Build history of the part. All positions in model axes, mm. Face numbers are marked on the shaded views. A direction names the side the tool comes from. Round coordinates to 2 decimals unless told otherwise and drop trailing zeros. Write each loop counter-clockwise with the first axis right and the second up, starting at its lowest first coordinate (ties: lowest second). Pieces come first, ordered by that corner, then holes. Notation, with made-up numbers: (-8, 17) -> (18, 17) arc R11 cw to (18, 31) -> close; hole circle Ø7 at (84, 26). An arc over 180 degrees is marked (long way). Return JSON: item names as keys, results as strings.
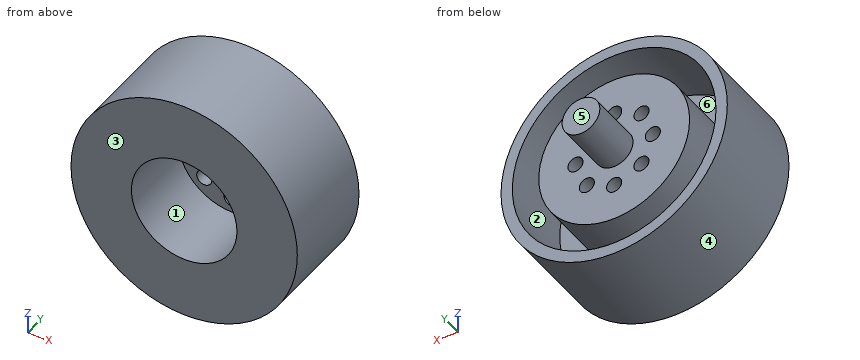
from build123d import *

# Parameters (mm, degrees)
F0_R      = 19.05
F1_DEPTH  = 16.51
F2_R      = 8.89
F4_DEPTH  = 12.7
F3_R      = 1.27
F5_DEPTH  = 25.4
F6_R      = 3.175
F7_DEPTH  = 12.7
F8_R      = 4.445
F9_DEPTH  = 0.635
F10_R     = 1.27
F11_DEPTH = 2.54
F12_R     = 0.508
F13_DEPTH = 1.016
F14_R     = 17.145
F14_R_2   = 12.7
F15_DEPTH = 12.7


with BuildPart() as f1:
    # F0 (on Front) → F1 (new body)
    with BuildSketch(Plane.XZ):
        Circle(F0_R)
    extrude(amount=-F1_DEPTH)

    # F2 (on face) → F4 (cut)
    with BuildSketch(Plane.XZ):
        Circle(F2_R)
    extrude(amount=-F4_DEPTH, mode=Mode.SUBTRACT)

    # F3 (on face) → F5 (cut)
    with BuildSketch(Plane.XZ):
        with Locations((0, 6.510976)):
            Circle(F3_R)
        with Locations((4.603955, 4.603955)):
            Circle(F3_R)
        with Locations((6.510976, 0)):
            Circle(F3_R)
        with Locations((4.603955, -4.603955)):
            Circle(F3_R)
        with Locations((0, -6.510976)):
            Circle(F3_R)
        with Locations((-4.603955, -4.603955)):
            Circle(F3_R)
        with Locations((-6.510976, 0)):
            Circle(F3_R)
        with Locations((-4.603955, 4.603955)):
            Circle(F3_R)
    extrude(amount=-F5_DEPTH, mode=Mode.SUBTRACT)

    # F6 (on face) → F7 (join)
    with BuildSketch(Plane.XZ.offset(-12.7)):
        Circle(F6_R)
    extrude(amount=-F7_DEPTH)

    # F8 (on face) → F9 (join)
    with BuildSketch(Plane.XZ.offset(-12.7)):
        Circle(F8_R)
    extrude(amount=F9_DEPTH)

    # F10 (on face) → F11 (join)
    with BuildSketch(Plane.XZ.offset(-12.065)):
        Circle(F10_R)
    extrude(amount=F11_DEPTH)

    # F12 (on face) → F13 (join)
    with BuildSketch(Plane.XZ.offset(-12.065)):
        with Locations((1.77372, 2.441316)):
            Circle(F12_R)
        with Locations((2.869939, 0.9325)):
            Circle(F12_R)
        with Locations((2.869939, -0.9325)):
            Circle(F12_R)
        with Locations((1.77372, -2.441316)):
            Circle(F12_R)
        with Locations((0, -3.017632)):
            Circle(F12_R)
        with Locations((-1.77372, -2.441316)):
            Circle(F12_R)
        with Locations((-2.869939, -0.9325)):
            Circle(F12_R)
        with Locations((-2.869939, 0.9325)):
            Circle(F12_R)
        with Locations((-1.77372, 2.441316)):
            Circle(F12_R)
        with Locations((0, 3.017632)):
            Circle(F12_R)
    extrude(amount=F13_DEPTH)

    # F14 (on face) → F15 (cut)
    with BuildSketch(Plane(origin=(0, 16.51, 0), x_dir=(-1, 0, 0), z_dir=(0, 1, 0))):
        Circle(F14_R)
        Circle(F14_R_2, mode=Mode.SUBTRACT)
    extrude(amount=-F15_DEPTH, mode=Mode.SUBTRACT)


solid = f1.part
Q1. Saw through at C-C on x = -11. List the corners of the cut face in (y, z), then the cut area to 3 significant figures.
Verdict:
{"outline": "(0, -15.55) -> (16.51, -15.55) -> (16.51, -13.15) -> (3.81, -13.15) -> (3.81, -6.35) -> (16.51, -6.35) -> (16.51, 6.35) -> (3.81, 6.35) -> (3.81, 13.15) -> (16.51, 13.15) -> (16.51, 15.55) -> (0, 15.55) -> close", "area": "341 mm²"}
Q2. Two-plate mould, pull along X, no slides. Class the marked faces 4, 5 and 6: +X half, -X half, draft (parallel to the pull), parting line (faces both ways), or undercut.
Verdict:
{"face 4": "parting line", "face 5": "draft", "face 6": "undercut"}
Q3. Pin check, flat tips, straight feed: pin 1 Ø12 at (x, z) = (-8, 15) entering from +Y; pin 2 Ø3 at (x, y) = (-12, 5.5) entering from -Z; pin 3 Ø1.1 at (x, z) = (-2, 2.5) entering from -Y; pin 4 Ø1.5 at (x, z) = (4.6, 4.6) entering from -Y. Stop position of each tip, or through.
Verdict:
{"pin 1": "stops at y = 16.51", "pin 2": "stops at z = -15.9", "pin 3": "stops at y = 11.05", "pin 4": "passes through"}
Q4. Wall check: L1, parallel to Z at x = 0, y = 9 (3 decimals); L2, parallel to Z at x = 0, y = 12.5 (3 decimals); L3, parallel to Z at x = -3.5, y = 4. Give the ranges that are in metal, low to high.
Verdict:
{"L1": "z = -19.05 to -17.145, -12.7 to -8.89, 8.89 to 12.7, 17.145 to 19.05", "L2": "z = -19.05 to -17.145, -12.7 to -8.89, -4.445 to 4.445, 8.89 to 12.7, 17.145 to 19.05", "L3": "z = -18.73 to -16.78, -12.21 to -8.17, 8.17 to 12.21, 16.78 to 18.73"}
Q5. Saw through at B-B on y = 16. Count the separate pieces of the cut face and the enclosed holes in it, then the cut area to 3 significant figures.
Verdict:
{"separate pieces": "2", "enclosed holes": "9", "area": "683 mm²"}
Q6. 3-axis set-ups, long thin cutter, end or side, ignore diameter. For the marked faces 1, 2 and 3: which of +Z, -Z, +X, -X, +Y, -Y reach the whole face in a straight line?
Verdict:
{"face 1": "-Y", "face 2": "+Y", "face 3": "+Z, -Z, +X, -X, -Y"}
Q7. Saw through at A-A on y = 10.5. List the corners of the cut face in (x, z) (3 decimals).
Verdict:
{"outline": "circle Ø38.1 at (0, 0); circle Ø25.4 at (0, 0); circle Ø2.54 at (0, 0); hole circle Ø34.29 at (0, 0); hole circle Ø17.78 at (0, 0)"}
